Input: part model. Units: mm. Frame: model coordinates. Face numbers are marked on the shaded views. A direction names the side the tool comes from. Coordinates: 2 decimals unless noted, no trailing zeros. Order: outer loops, then holes, each group sorted by start corner. A loop starts at its lowest first (then second) coordinate and runs counter-clockwise, first axis right, second up.
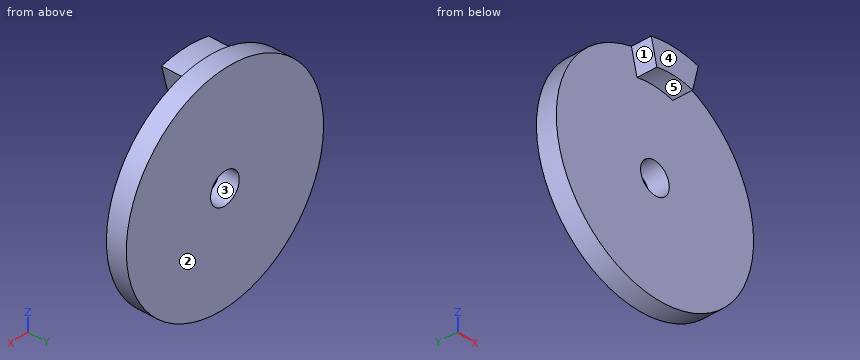
from build123d import *
from build123d.topology import SkipClean

# Parameters (mm, degrees)
SKETCH2_R           = 34.925
SKETCH2_R_2         = 5.08
BOSS_EXTRUDE1_DEPTH = 6.35
BOSS_EXTRUDE2_START = 6.35
BOSS_EXTRUDE2_DEPTH = 6.35


with BuildPart() as part:
    # Sketch2 → Boss-Extrude1 (new body)
    with BuildSketch(Plane(origin=(0, 0, 0), x_dir=(1, 0, 0), z_dir=(0, 1, 0))):
        with Locations(Location((0, 0, 0), (0, 0, 270))):
            Circle(SKETCH2_R)
        with Locations(Location((0, 0, 0), (0, 0, 270))):
            Circle(SKETCH2_R_2, mode=Mode.SUBTRACT)
    extrude(amount=BOSS_EXTRUDE1_DEPTH)

    # Sketch3 → Boss-Extrude2 (add)
    with SkipClean():  # the faces are left unmerged after this step: merging them gives an invalid solid
        with BuildSketch(Plane.XZ.offset(BOSS_EXTRUDE2_START)):
            with BuildLine():
                Line((6.35, 25.903019129), (8.31547619, 33.920620288))
                ThreePointArc((8.31547619, 33.920620288), (0, 34.925), (-8.31547619, 33.920620288))
                Line((-8.31547619, 33.920620288), (-6.35, 25.903019129))
                ThreePointArc((-6.35, 25.903019129), (0, 26.67), (6.35, 25.903019129))
            make_face()
        extrude(amount=-BOSS_EXTRUDE2_DEPTH)


solid = part.part
Item 1: Draft query along Z for the marked faces 3, 4 and 5. Return one class per face: pulls with the +Z half, pulls with the -Z half, needs draft (parallel to the pull), parting line crosses it, or undercut.
Response values:
face 3: undercut
face 4: needs draft
face 5: pulls with the -Z half
Item 2: Cut plane D-D on y = -3.5. Return loops of the section in (x, z) (3 decimals), then the cut area to 3 significant figures.
Response values:
outline: (-8.315, 33.921) - (-6.35, 25.903) arc R26.67 cw to (6.35, 25.903) - (8.315, 33.921) arc R34.925 ccw to start
area: 122 mm2
Item 3: Cut plane A-A on x = 0. Return loops of the section in (y, z) (3 decimals), then the cut area to 3 significant figures.
Response values:
outline: (-6.35, 26.67) - (0, 26.67) - (0, 5.08) - (6.35, 5.08) - (6.35, 34.925) - (-6.35, 34.925) - close; (0, -34.925) - (6.35, -34.925) - (6.35, -5.08) - (0, -5.08) - close
area: 431 mm2
Item 4: Cut plane B-B on z = 0. Return loops of the section in (x, y) (3 decimals), then the cut area to 3 significant figures.
Response values:
outline: (-34.925, 0) - (-5.08, 0) - (-5.08, 6.35) - (-34.925, 6.35) - close; (5.08, 0) - (34.925, 0) - (34.925, 6.35) - (5.08, 6.35) - close
area: 379 mm2
Item 5: Ray query, probe 1 along X at (y, z) = (2, 0) (3 decimals); probe 2 along Y at (x, z) = (18.5, -10.5); probe 3 along Z at (x, y) = (-1, -5.25). Return the intervals inside material, ascending.
Response values:
probe 1: x = -34.925 to -5.08, 5.08 to 34.925
probe 2: y = 0 to 6.35
probe 3: z = 26.65 to 34.91
Item 6: Pin query (flat end, axial travel): pin 1 Ø6 at (x, z) = (-2.5, 7) entering from -Y; pin 2 Ø1.5 at (y, z) = (-0.5, -24.5) entering from -X; pin 3 Ø1 at (x, y) = (-6.5, 0) entering from +Z; pin 4 Ø9 at (x, z) = (0, 0) entering from +Y. Return the tip coordinate at first contact, or that it passes through.
Response values:
pin 1: stops at y = 0
pin 2: stops at x = -25.43
pin 3: stops at z = 34.41
pin 4: passes through
Item 7: Cut plane C-C on y = 5.25. Return loops of the section in (x, z) (3 decimals).
Response values:
outline: circle Ø69.85 at (0, 0); hole circle Ø10.16 at (0, 0)
Item 8: Access query for the marked faces 1 and 2. Directions: +Z, -Z, +X, -X, +Y, -Y. A direction counts if a zero-diameter tool reaches every point of the face in a straight line with its end or side. Return the directions, or none.
Response values:
face 1: -Z, -X, -Y
face 2: +Z, -Z, +X, -X, +Y
